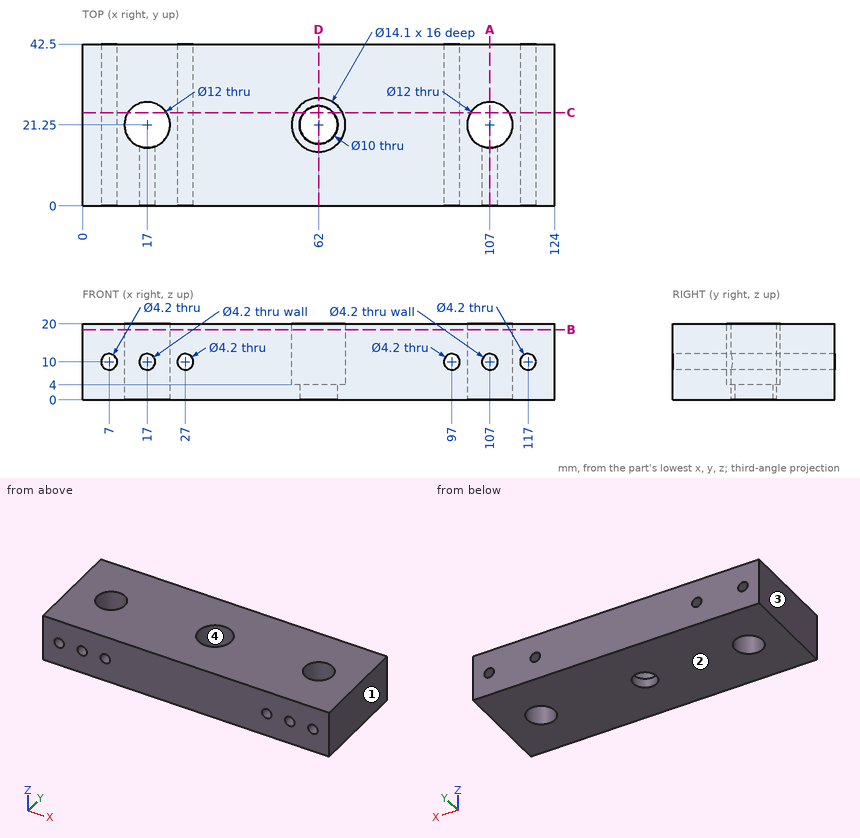
Check sheet for the drawn part. Datum: minimum x, y, z corner. Units: mm. Give positions to 0.01 mm unless a question says otherwise; leave off trailing zeros. Loops run counter-clockwise (first coordinate to the right, second up) from the corner with the lowest first, then second, coordinate; pieces in that order, holes last. Notation, with made-up numbers: M -40,20 L 12,20 A23 cw 12,37 Z; hole C 72.5,62.25 d8. An arc over 180 degrees is marked long. Answer as CSV lines item,"result".
Item 1: Sectioned sample at B-B, the plane z = 18.5. Enter the section's corners in (x, y).
Reply:
outline,"M 0,0 L 124,0 L 124,42.5 L 0,42.5 Z; hole C 17,21.25 d12; hole C 62,21.25 d14.1; hole C 107,21.25 d12"
Item 2: Sectioned sample at D-D, the plane x = 62. Enter the section's corners in (y, z), then the cut area to 3 significant figures.
Reply:
outline,"M 0,0 L 16.25,0 L 16.25,4 L 14.2,4 L 14.2,20 L 0,20 Z; M 26.25,0 L 42.5,0 L 42.5,20 L 28.3,20 L 28.3,4 L 26.25,4 Z"
area,"584 mm^2"
Item 3: Depth check by flat-ended pin: pin 1 Ø2.5 at (x, z) = (107, 10) entering from -Y; pin 2 Ø4 at (x, y) = (63.5, 22) entering from +Z; pin 3 Ø11.5 at (x, y) = (62, 21.25) entering from +Z. Enter the tip coordinate at first touch or a pass-through.
Reply:
pin 1,"y = 27.12"
pin 2,"through"
pin 3,"z = 4"
Item 4: Scan lines: L1, parallel to X at y = 25.5, z = 15.25; L2, parallel to X at y = 16, z = 19; L3, parallel to Z at x = 117, y = 21. Record each from-to range of solid material in increasing order.
Reply:
L1,"0 to 12.76, 21.24 to 56.38, 67.62 to 102.76, 111.24 to 124"
L2,"0 to 14.1, 19.9 to 57.29, 66.71 to 104.1, 109.9 to 124"
L3,"0 to 7.9, 12.1 to 20"
Item 5: Sectioned sample at C-C, the plane y = 24.5. Enter the section's corners in (x, z), then the cut area to 3 significant figures.
Reply:
outline,"M 0,0 L 11.96,0 L 11.96,20 L 0,20 Z; M 22.04,0 L 58.2,0 L 58.2,4 L 55.74,4 L 55.74,20 L 22.04,20 Z; M 65.8,0 L 101.96,0 L 101.96,20 L 68.26,20 L 68.26,4 L 65.8,4 Z; M 112.04,0 L 124,0 L 124,20 L 112.04,20 Z; hole C 7,10 d4.2; hole C 27,10 d4.2; hole C 97,10 d4.2; hole C 117,10 d4.2"
area,"1,790 mm^2"
Item 6: Draft check along X on the marked faces 1, 2, 3 and 4. Enter one of: pulls with the +X half, pulls with the -X half, needs draft (parallel to the pull), parting line crosses it, or undercut.
Reply:
face 1,"pulls with the +X half"
face 2,"needs draft"
face 3,"pulls with the -X half"
face 4,"undercut"
Item 7: Sectioned sample at A-A, the plane x = 107. Enter the section's corners in (y, z).
Reply:
outline,"M 0,0 L 15.25,0 L 15.25,7.9 L 0,7.9 Z; M 0,12.1 L 15.25,12.1 L 15.25,20 L 0,20 Z; M 27.25,0 L 42.5,0 L 42.5,20 L 27.25,20 Z"
